from build123d import *

# Parameters (mm, degrees)
F0_R     = 12
F1_DEPTH = 1.5
F2_DEPTH = 2
F3_DEPTH = 9.98
F4_DEPTH = 1


with BuildPart() as f1:
    # F0 (on Top) → F1 (new body)
    with BuildSketch(Plane.XY):
        Circle(F0_R)
        with BuildLine():
            ThreePointArc((4.0121757808, 4.461215698), (4.6995946202, 3.7301220363), (5.2555497929, 2.8946841579))
            ThreePointArc((5.2555497929, 2.8946841579), (5.810907793, 1.4944399022), (6, 0))
            ThreePointArc((6, 0), (-5.4805590356, -2.4420222476), (4.0121757808, 4.461215698))
        make_face(mode=Mode.SUBTRACT)
        with BuildLine():
            ThreePointArc((2.6747838539, 2.9741437986), (3.1330630801, 2.4867480242), (3.503699862, 1.9297894386))
            Line((3.503699862, 1.9297894386), (5.2555497929, 2.8946841579))
            ThreePointArc((5.2555497929, 2.8946841579), (4.6995946202, 3.7301220363), (4.0121757808, 4.461215698))
            Line((4.0121757808, 4.461215698), (2.6747838539, 2.9741437986))
        make_face()
        with BuildLine():
            Line((5.2555497929, 2.8946841579), (3.503699862, 1.9297894386))
            ThreePointArc((3.503699862, 1.9297894386), (3.8739385287, 0.9962932681), (4, 0))
            ThreePointArc((4, 0), (-3.6537060237, -1.6280148317), (2.6747838539, 2.9741437986))
            Line((2.6747838539, 2.9741437986), (4.0121757808, 4.461215698))
            ThreePointArc((4.0121757808, 4.461215698), (-5.4805590356, -2.4420222476), (6, 0))
            ThreePointArc((6, 0), (5.810907793, 1.4944399022), (5.2555497929, 2.8946841579))
        make_face()
        with BuildLine():
            ThreePointArc((2.0060878904, 2.230607849), (2.3497973101, 1.8650610182), (2.6277748965, 1.447342079))
            Line((2.6277748965, 1.447342079), (2.715367393, 1.4955868149))
            ThreePointArc((2.715367393, 1.4955868149), (2.4281238871, 1.9272297188), (2.0729574868, 2.304961444))
            Line((2.0729574868, 2.304961444), (2.0060878904, 2.230607849))
        make_face()
        with BuildLine():
            ThreePointArc((2.6277748965, 1.447342079), (2.9054538965, 0.7472199511), (3, 0))
            ThreePointArc((3, 0), (-2.7402795178, -1.2210111238), (2.0060878904, 2.230607849))
            Line((2.0060878904, 2.230607849), (2.0729574868, 2.304961444))
            ThreePointArc((2.0729574868, 2.304961444), (-2.8316221684, -1.2617114946), (3.1, 0))
            ThreePointArc((3.1, 0), (3.0023023597, 0.7721272828), (2.715367393, 1.4955868149))
            Line((2.715367393, 1.4955868149), (2.6277748965, 1.447342079))
        make_face()
        with BuildLine():
            Line((0, 0), (2.6277748965, 1.447342079))
            ThreePointArc((2.6277748965, 1.447342079), (2.3497973101, 1.8650610182), (2.0060878904, 2.230607849))
            Line((2.0060878904, 2.230607849), (0, 0))
        make_face()
        with BuildLine():
            ThreePointArc((2.0060878904, 2.230607849), (-2.7402795178, -1.2210111238), (3, 0))
            ThreePointArc((3, 0), (2.9054538965, 0.7472199511), (2.6277748965, 1.447342079))
            Line((2.6277748965, 1.447342079), (0, 0))
            Line((0, 0), (2.0060878904, 2.230607849))
        make_face()
        with BuildLine():
            Line((3.503699862, 1.9297894386), (2.715367393, 1.4955868149))
            ThreePointArc((2.715367393, 1.4955868149), (3.0023023597, 0.7721272828), (3.1, 0))
            ThreePointArc((3.1, 0), (-2.8316221684, -1.2617114946), (2.0729574868, 2.304961444))
            Line((2.0729574868, 2.304961444), (2.6747838539, 2.9741437986))
            ThreePointArc((2.6747838539, 2.9741437986), (-3.6537060237, -1.6280148317), (4, 0))
            ThreePointArc((4, 0), (3.8739385287, 0.9962932681), (3.503699862, 1.9297894386))
        make_face()
        with BuildLine():
            ThreePointArc((2.0729574868, 2.304961444), (2.4281238871, 1.9272297188), (2.715367393, 1.4955868149))
            Line((2.715367393, 1.4955868149), (3.503699862, 1.9297894386))
            ThreePointArc((3.503699862, 1.9297894386), (3.1330630801, 2.4867480242), (2.6747838539, 2.9741437986))
            Line((2.6747838539, 2.9741437986), (2.0729574868, 2.304961444))
        make_face()
    extrude(amount=F1_DEPTH)



with BuildPart() as f2:
    # F0 (on Top) → F2 (new body)
    with BuildSketch(Plane.XY):
        with BuildLine():
            ThreePointArc((2.6747838539, 2.9741437986), (3.1330630801, 2.4867480242), (3.503699862, 1.9297894386))
            Line((3.503699862, 1.9297894386), (5.2555497929, 2.8946841579))
            ThreePointArc((5.2555497929, 2.8946841579), (4.6995946202, 3.7301220363), (4.0121757808, 4.461215698))
            Line((4.0121757808, 4.461215698), (2.6747838539, 2.9741437986))
        make_face()
        with BuildLine():
            Line((5.2555497929, 2.8946841579), (3.503699862, 1.9297894386))
            ThreePointArc((3.503699862, 1.9297894386), (3.8739385287, 0.9962932681), (4, 0))
            ThreePointArc((4, 0), (-3.6537060237, -1.6280148317), (2.6747838539, 2.9741437986))
            Line((2.6747838539, 2.9741437986), (4.0121757808, 4.461215698))
            ThreePointArc((4.0121757808, 4.461215698), (-5.4805590356, -2.4420222476), (6, 0))
            ThreePointArc((6, 0), (5.810907793, 1.4944399022), (5.2555497929, 2.8946841579))
        make_face()
        with BuildLine():
            Line((3.503699862, 1.9297894386), (2.715367393, 1.4955868149))
            ThreePointArc((2.715367393, 1.4955868149), (3.0023023597, 0.7721272828), (3.1, 0))
            ThreePointArc((3.1, 0), (-2.8316221684, -1.2617114946), (2.0729574868, 2.304961444))
            Line((2.0729574868, 2.304961444), (2.6747838539, 2.9741437986))
            ThreePointArc((2.6747838539, 2.9741437986), (-3.6537060237, -1.6280148317), (4, 0))
            ThreePointArc((4, 0), (3.8739385287, 0.9962932681), (3.503699862, 1.9297894386))
        make_face()
        with BuildLine():
            ThreePointArc((2.0729574868, 2.304961444), (2.4281238871, 1.9272297188), (2.715367393, 1.4955868149))
            Line((2.715367393, 1.4955868149), (3.503699862, 1.9297894386))
            ThreePointArc((3.503699862, 1.9297894386), (3.1330630801, 2.4867480242), (2.6747838539, 2.9741437986))
            Line((2.6747838539, 2.9741437986), (2.0729574868, 2.304961444))
        make_face()
    extrude(amount=F2_DEPTH)


with BuildPart() as f1_1:
    add(f1.part)

    add(f2.part)  # F3 merges F2
    # F0 (on Top) → F3 (join)
    with BuildSketch(Plane.XY):
        with BuildLine():
            ThreePointArc((2.6277748965, 1.447342079), (2.9054538965, 0.7472199511), (3, 0))
            ThreePointArc((3, 0), (-2.7402795178, -1.2210111238), (2.0060878904, 2.230607849))
            Line((2.0060878904, 2.230607849), (2.0729574868, 2.304961444))
            ThreePointArc((2.0729574868, 2.304961444), (-2.8316221684, -1.2617114946), (3.1, 0))
            ThreePointArc((3.1, 0), (3.0023023597, 0.7721272828), (2.715367393, 1.4955868149))
            Line((2.715367393, 1.4955868149), (2.6277748965, 1.447342079))
        make_face()
        with BuildLine():
            Line((3.503699862, 1.9297894386), (2.715367393, 1.4955868149))
            ThreePointArc((2.715367393, 1.4955868149), (3.0023023597, 0.7721272828), (3.1, 0))
            ThreePointArc((3.1, 0), (-2.8316221684, -1.2617114946), (2.0729574868, 2.304961444))
            Line((2.0729574868, 2.304961444), (2.6747838539, 2.9741437986))
            ThreePointArc((2.6747838539, 2.9741437986), (-3.6537060237, -1.6280148317), (4, 0))
            ThreePointArc((4, 0), (3.8739385287, 0.9962932681), (3.503699862, 1.9297894386))
        make_face()
    extrude(amount=F3_DEPTH)


with BuildPart() as f4:
    # F0 (on Top) → F4 (new body)
    with BuildSketch(Plane.XY):
        with BuildLine():
            ThreePointArc((2.6277748965, 1.447342079), (2.9054538965, 0.7472199511), (3, 0))
            ThreePointArc((3, 0), (-2.7402795178, -1.2210111238), (2.0060878904, 2.230607849))
            Line((2.0060878904, 2.230607849), (2.0729574868, 2.304961444))
            ThreePointArc((2.0729574868, 2.304961444), (-2.8316221684, -1.2617114946), (3.1, 0))
            ThreePointArc((3.1, 0), (3.0023023597, 0.7721272828), (2.715367393, 1.4955868149))
            Line((2.715367393, 1.4955868149), (2.6277748965, 1.447342079))
        make_face()
    extrude(amount=F4_DEPTH)


with BuildPart() as f4_1:
    # F5: moved
    add(f4.part.moved(Location((0, 0, 6))))


with BuildPart() as f1_2:
    add(f1_1.part)

    # F6: cut F4
    add(f4_1.part, mode=Mode.SUBTRACT)


solid = f1_2.part
Work out the finished part from the listing and answer in its coordinate system (mm). A direction names the side the tool comes from. Round coordinates to 2 decimals unless told otherwise and drop trailing zeros. Write each loop counter-clockwise with the first axis right and the second up, starting at its lowest first coordinate (ties: lowest second). Pieces come first, ordered by that corner, then holes. Notation, with made-up numbers: (55, 2.25) -> (90, 2.25) arc R31 cw to (90, 33.25) -> close; hole circle Ø6 at (50.5, 10). An arc over 180 degrees is marked (long way). Answer as CSV lines item,"result". Start each with the question number.
(1) The part is cut by section A-A, the plane z = 2.5. Give the vertices of the cut face in (x, y), then the cut area to 3 significant figures.
(2) The part is cut by section D-D, the plane y = 9. Give the vertices of the cut face in (x, z), then the cut area to 3 significant figures.
(3) The part is cut by section C-C, the plane z = 6.5. Give the vertices of the cut face in (x, y).
(4) The part is cut by section B-B, the plane x = 0. Give the vertices of the cut face in (y, z), then the cut area to 3 significant figures.
(5) Find the intervals of material crossed by probe 1 along X at (y, z) = (0, 6.2); probe 2 along Y at (x, z) = (0, 2.95); probe 3 along Z at (x, y) = (2.25, 7.25), in increasing order.
(6) Each of these flat-tipped pins is pushed along its axis until it touches: pin 1 (1.5 mm diameter, centred on x = -1.5, y = 9.5, fed in from +Z); pin 2 (5 mm diameter, centred on x = -0.5, z = 5.5, fed in from +Y). Where does it stop, or does it pass through?
(7) A tool of negligible diameter and unlimited length cuts with its end or side. For faces 1 (the flat face through (-3, -1, 9.98)), 2 (the flat face through (-6, -2, 1.5)), from which of +Z, -Z, +X, -X, +Y, -Y can it reach the whole face along a straight path? Write none if from no direction.
(8) The mould has two halves that part along X. Classify faces 3 (the flat face through (0, 0, 1.5)), 4 (the cylindrical face through (-11.99, 0.53, 0.74)), 5 (the flat face through (0, 0, 0)): +X half, -X half, draft (parallel to the pull), parting line (faces both ways), or undercut.
Output values:
1,outline,"(2.01, 2.23) -> (2.67, 2.97) arc R4 ccw (long way) to (3.5, 1.93) -> (2.63, 1.45) arc R3 cw (long way) to start"
1,area,"20.8 mm²"
2,outline,"(-7.94, 0) -> (7.94, 0) -> (7.94, 1.5) -> (-7.94, 1.5) -> close"
2,area,"23.8 mm²"
3,outline,"(2.07, 2.3) -> (2.67, 2.97) arc R4 ccw (long way) to (3.5, 1.93) -> (2.72, 1.5) arc R3.1 cw (long way) to start"
4,outline,"(-12, 0) -> (12, 0) -> (12, 1.5) -> (6, 1.5) -> (6, 2) -> (4, 2) -> (4, 9.98) -> (3, 9.98) -> (3, 7) -> (3.1, 7) -> (3.1, 6) -> (3, 6) -> (3, 1.5) -> (-3, 1.5) -> (-3, 6) -> (-3.1, 6) -> (-3.1, 7) -> (-3, 7) -> (-3, 9.98) -> (-4, 9.98) -> (-4, 2) -> (-6, 2) -> (-6, 1.5) -> (-12, 1.5) -> close"
4,area,"54.8 mm²"
5,probe 1,"x = -4 to -3.1, 3.1 to 4"
5,probe 2,"y = -4 to -3, 3 to 4"
5,probe 3,"z = 0 to 1.5"
6,pin 1,"stops at z = 1.5"
6,pin 2,"stops at y = 4"
7,face 1,"+Z, +X, -X, +Y, -Y"
7,face 2,"+Z"
8,face 3,"undercut"
8,face 4,"parting line"
8,face 5,"draft"
